Work out the finished part from the listing and answer in its coordinate system (mm). A direction names the side the tool comes from. Round coordinates to 2 decimals unless told otherwise and drop trailing zeros. Write each loop counter-clockwise with the first axis right and the second up, starting at its lowest first coordinate (ties: lowest second). Pieces come first, ordered by that corner, then holes. Notation, with made-up numbers: M -28,44.5 L 29,44.5 A18 ccw 29,50.5 Z; hole C 73,43 d9. An arc over 180 degrees is marked long. One line per item, written item: value. Start each with the question number.
Q1. The mould has two halves that part along Z. Classify faces 5 (the cylindrical face through (7.2, 13.5, -5.6)), 6 (the flat face through (12, 1, -34)), 7 (the flat face through (2, 7, 0)): released by +Z, released by -Z, zero draft, split by the parting line, or undercut.
Q2. Consider probe 1 along Z at (x, y) = (6, 12.8); probe 2 along Z at (x, y) = (6, 1.6); probe 3 along Y at (x, z) = (9.25, -30). Determine where each line is inside the solid, lowest interval first.
Q3. Find section B-B (z = -53). Write down the section's boundary in (x, y).
Q4. A tool of negligible diameter and unlimited length cuts with its end or side. For faces 1 (the cylindrical face through (5.93, 1.52, -13.5)), 2 (the flat face through (12, 13, -34)), 3 (the flat face through (8, 12, -34)), 4 (the cylindrical face through (6.766, 13.479, -62.153)), from which of +Z, -Z, +X, -X, +Y, -Y can it reach the whole face along a straight path? Write none if from no direction.
Q5. Given pin 1 Ø2.5 at (x, z) = (6, -53) entering from -Y; pin 2 Ø4.5 at (y, z) = (8, -39.5) entering from +X; pin 3 Ø1 at (x, y) = (6.5, 4) entering from +Z, each flat-ended and moving along its own axis, determine where each tip first touches the part or whether it passes through.
Q6. Find section A-A (x = 10.75). Write down the section's boundary in (y, z).
Q7. Find section C-C (x = 6). Write down the section's boundary in (y, z), and give its area (3 significant figures).
Q8. Find section D-D (z = -19). Write down the section's boundary in (x, y).
Autodesk Inventor part; units mm, degrees
ref_plane "YZ Plane" through (0, 0, 0) normal (1, 0, 0) x (0, 1, 0)
ref_plane "XZ Plane" through (0, 0, 0) normal (0, 1, 0) x (-1, 0, 0)
ref_plane "XY Plane" through (0, 0, 0) normal (0, 0, 1) x (1, 0, 0)
sketch "Sketch1" plane through (0, 0, 0) normal (0, 1, 0) x (-1, 0, 0)
  line L0 (0, 0) -> (-12, 0)
  line L1 (-12, 0) -> (-12, -68)
  line L2 (-12, -68) -> (0, -68)
  line L3 (0, -68) -> (0, 0)
  dimension "d0" = 12
  dimension "d1" = 68
extrude "Extrusion1" add sketch "Sketch1" along normal blind 15
sketch "Sketch4" plane through (12, 0, 0) normal (1, 0, 0) x (0, 0, -1)
  line L0 (0, 0) -> (0, 15)
  line L1 (0, 3) -> (68, 3)
  line L2 (68, 3) -> (68, 12)
  line L3 (68, 12) -> (0, 12)
  line L4 (0, 12) -> (0, 3)
  line L5 (0, 0) -> (68, 0)
  dimension "d30" = 68
  dimension "d31" = 9
  dimension "d32" = 3
extrude "Extrusion2" cut sketch "Sketch4" against normal blind 9
sketch "Sketch2" plane through (0, 15, 0) normal (0, 1, 0) x (1, 0, 0)
  circle A0 centre (6, 64) radius 2
  circle A1 centre (6, 4) radius 2
  line L0 (0, 68) -> (0, 0)
  line L1 (12, 68) -> (0, 68)
  line L2 (0, 0) -> (12, 0)
  dimension "d4" = 4
  dimension "d5" = 4
  dimension "d6" = 6
  dimension "d7" = 6
  dimension "d8" = 4
  dimension "d9" = 4
hole "Hole1" at (6, 15, -4) at (6, 15, -64) direction (0, -1, 0) diameter 4 depth 3 tip angle 118
sketch "Sketch3" plane through (0, 0, 0) normal (0, -1, 0) x (1, 0, 0)
  circle A0 centre (6, -15) radius 1.5
  circle A1 centre (6, -53) radius 1.5
  line L0 (0, -68) -> (0, 0)
  line L1 (0, 0) -> (12, 0)
  line L2 (12, -68) -> (0, -68)
  dimension "d17" = 3
  dimension "d18" = 3
  dimension "d19" = 6
  dimension "d20" = 6
  dimension "d21" = 15
  dimension "d22" = 15
hole "Hole2" at (6, 0, -53) at (6, 0, -15) direction (0, 1, 0) diameter 3 depth 3 tip angle 118
thread "Thread1"
thread "Thread2"
thread "Thread3"
thread "Thread4"
properties part number "sensor3_lock" material "Aluminum 6061"
The answers:
1. face 5: undercut
1. face 6: zero draft
1. face 7: released by +Z
2. probe 1: -68 to -66, -62 to -6, -2 to 0
2. probe 2: -68 to -54.5, -51.5 to -16.5, -13.5 to 0
2. probe 3: 0 to 3, 12 to 15
3. outline: M 0,0 L 4.5,0 L 4.5,3 L 3,3 L 3,12 L 12,12 L 12,15 L 0,15 Z; M 7.5,0 L 12,0 L 12,3 L 7.5,3 Z
4. face 1: -Y
4. face 2: +Z, -Z, +X, +Y, -Y
4. face 3: +Z, -Z, +X
4. face 4: +Y
5. pin 1: y = 12
5. pin 2: x = 3
5. pin 3: through
6. outline: M 0,-68 L 3,-68 L 3,0 L 0,0 Z; M 12,-68 L 15,-68 L 15,0 L 12,0 Z
7. outline: M 0,-68 L 3,-68 L 3,-54.5 L 0,-54.5 Z; M 0,-51.5 L 3,-51.5 L 3,-16.5 L 0,-16.5 Z; M 0,-13.5 L 3,-13.5 L 3,0 L 0,0 Z; M 12,-68 L 15,-68 L 15,-66 L 12,-66 Z; M 12,-62 L 15,-62 L 15,-6 L 12,-6 Z; M 12,-2 L 15,-2 L 15,0 L 12,0 Z
7. area: 366 mm2
8. outline: M 0,0 L 12,0 L 12,3 L 3,3 L 3,12 L 12,12 L 12,15 L 0,15 Z
